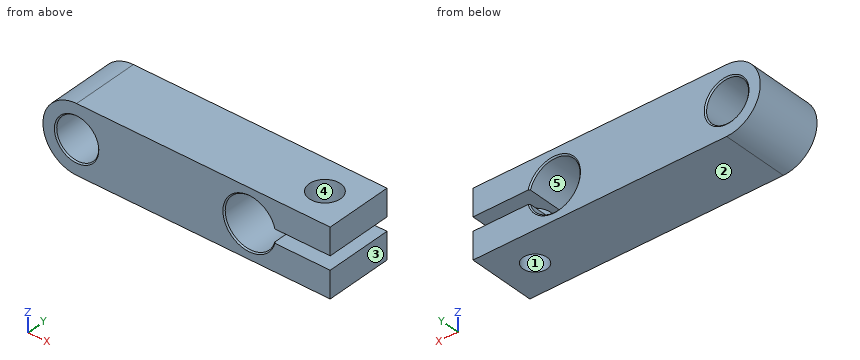
from build123d import *
from OCP.BRepFilletAPI import BRepFilletAPI_MakeChamfer

# Parameters (mm, degrees)
SKETCH1_R                  = 1.9812
SKETCH1_R_2                = 2.38125
BOSS_EXTRUDE1_DEPTH        = 6.35
SKETCH2_W                  = 7.62
SKETCH2_H                  = 1.27
CUT_EXTRUDE1_DEPTH         = 26.532761738
CHAMFER1_SIZE              = 0.127
CHAMFER1_SIZE2             = 0.110399416
F_4_40_TAPPED_HOLE1_REACH  = 27.533
F_4_40_TAPPED_HOLE1_BORE_R = 1.1303
SKETCH5_R                  = 1.4732
CUT_EXTRUDE2_DEPTH         = 2.54


with BuildPart() as part:
    # Sketch1 → Boss-Extrude1 (new body)
    with BuildSketch(Plane(origin=(0, 0, 0), x_dir=(1, 0, 0), z_dir=(0, 1, 0))):
        with BuildLine():
            Line((0, 0), (23.9014, 0))
            Line((23.9014, 0), (23.9014, 6.35))
            Line((23.9014, 6.35), (0, 6.35))
            ThreePointArc((0, 6.35), (-3.175, 3.175), (0, 0))
        make_face()
        with Locations(Location((0, 3.175, 0), (0, 0, 270))):
            Circle(SKETCH1_R, mode=Mode.SUBTRACT)
        with Locations(Location((16.2814, 3.175, 0), (0, 0, 270))):
            Circle(SKETCH1_R_2, mode=Mode.SUBTRACT)
    extrude(amount=BOSS_EXTRUDE1_DEPTH)

    # Sketch2 → Cut-Extrude1 (cut, through all)
    with BuildSketch(Plane(origin=(0, 6.35, 0), x_dir=(1, 0, 0), z_dir=(0, 1, 0))):
        with Locations((20.0914, 3.175)):
            Rectangle(SKETCH2_W, SKETCH2_H)
    extrude(amount=-CUT_EXTRUDE1_DEPTH, mode=Mode.SUBTRACT)

    # Chamfer1: one chamfer whose edges measure the first distance from different faces: ONE call of the kernel's chamfer builder (chamfer() names one face for all edges)
    chamfer1_edges_1 = [part.edges().sort_by_distance(p)[0] for p in [
        (0, 0, -5.1562),
    ]]
    chamfer1_side_1 = [part.faces().sort_by_distance(p)[0] for p in [
        (0, 3.175, -5.1562),
    ]]
    chamfer1_edges_2 = [part.edges().sort_by_distance(p)[0] for p in [
        (0, 6.35, -5.1562),
        (13.90015, 6.35, -3.175),
    ]]
    chamfer1_side_2 = [part.faces().sort_by_distance(p)[0] for p in [
        (10.400868542, 6.35, -3.175),
    ]]
    chamfer1_edges_3 = [part.edges().sort_by_distance(p)[0] for p in [
        (13.90015, 0, -3.175),
    ]]
    chamfer1_side_3 = [part.faces().sort_by_distance(p)[0] for p in [
        (13.90015, 3.175, -3.175),
    ]]
    chamfer1 = BRepFilletAPI_MakeChamfer(part.part.solid().wrapped)
    for e in chamfer1_edges_1:
        chamfer1.Add(CHAMFER1_SIZE, CHAMFER1_SIZE2, e.wrapped, chamfer1_side_1[0].wrapped)  # the first distance lies on this face
    for e in chamfer1_edges_2:
        chamfer1.Add(CHAMFER1_SIZE, CHAMFER1_SIZE2, e.wrapped, chamfer1_side_2[0].wrapped)  # the first distance lies on this face
    for e in chamfer1_edges_3:
        chamfer1.Add(CHAMFER1_SIZE, CHAMFER1_SIZE2, e.wrapped, chamfer1_side_3[0].wrapped)  # the first distance lies on this face
    add(Compound.cast(chamfer1.Shape()), mode=Mode.REPLACE)

    # #4-40 Tapped Hole1 bore → #4-40 Tapped Hole1 (cut, up to next)
    with BuildSketch(Plane(origin=(0, 0, -6.35), x_dir=(-1, 0, 0), z_dir=(0, 0, -1)), mode=Mode.PRIVATE) as f_4_40_tapped_hole1_sk1:
        with Locations((-20.7264, 3.175)):
            Circle(F_4_40_TAPPED_HOLE1_BORE_R)
    f_4_40_tapped_hole1_tool1 = extrude(f_4_40_tapped_hole1_sk1.sketch, amount=-F_4_40_TAPPED_HOLE1_REACH, mode=Mode.PRIVATE) & part.part
    add(f_4_40_tapped_hole1_tool1.solids().sort_by_distance((20.7264, 3.175, -6.35))[0], mode=Mode.SUBTRACT)

    # Sketch5 → Cut-Extrude2 (cut)
    with BuildSketch(Plane.XY):
        with Locations((20.7264, 3.175)):
            Circle(SKETCH5_R)
    extrude(amount=-CUT_EXTRUDE2_DEPTH, mode=Mode.SUBTRACT)


solid = part.part
CAD build for the part. Positions are in the model's coordinates, mm. Face numbers are marked on the shaded views. A direction names the side the tool comes from. Coordinates: 2 decimals unless noted, no trailing zeros. Write each loop counter-clockwise with the first axis right and the second up, starting at its lowest first coordinate (ties: lowest second). Pieces come first, ordered by that corner, then holes. Notation, with made-up numbers: M 13,-34 L 37,-34 A31 cw 37,-6 Z; hole C 6.5,38 d1. An arc over 180 degrees is marked long. Answer as a JSON object with one key per item and string values. Group by question number.
1) Mould opens along X. For the marked faces 1, 2 and 3 say: +X half, -X half, draft (parallel to the pull), parting line (faces both ways), or undercut.
2) Wall check: line 1 (X direction, y = 3.25, z = -4.5); line 2 (Z direction, x = 19, y = 5.5); line 3 (X direction, y = 4.75, z = -4). Give the ranges that are in metal, low to high. Write a range as from..to.
3) Saw through at C-C (y = 4). Give the number of separate pieces and of enclosed holes in the cut face, plus the area to 3 significant figures.
4) Pin check, flat tips, straight feed: pin 1 Ø3 at (y, z) = (3, -3) entering from +X; pin 2 Ø1.8 at (x, y) = (20.73, 3.18) entering from -Z. Stop position of each tip, or through.
5) Tool access for the marked faces 4 and 5: list every direction of +Z, -Z, +X, -X, +Y, -Y with a clear straight run to the whole face (end or side of a thin tool).
6) Saw through at B-B (x = 20). Write the cut outline in (y, z), plus the area to 3 significant figures.
Values follow:
{
 "1": {"face 1": "undercut", "face 2": "draft", "face 3": "+X half"},
 "2": {"line 1": "x = -2.89..-1.47, 1.47..14.3, 18.26..19.6, 21.85..23.9", "line 2": "z = -6.35..-3.81, -2.54..0", "line 3": "x = -3.07..-1.8, 1.8..14.05, 18.52..23.9"},
 "3": {"separate pieces": "3", "enclosed holes": "1", "area": "121 mm2"},
 "4": {"pin 1": "stops at x = 23.9", "pin 2": "passes through"},
 "5": {"face 4": "+Z", "face 5": "+Y, -Y"},
 "6": {"outline": "M 0,-6.35 L 2.31,-6.35 L 2.31,-3.81 L 0,-3.81 Z; M 0,-2.54 L 1.89,-2.54 L 1.89,0 L 0,0 Z; M 4.04,-6.35 L 6.35,-6.35 L 6.35,-3.81 L 4.04,-3.81 Z; M 4.46,-2.54 L 6.35,-2.54 L 6.35,0 L 4.46,0 Z", "area": "21.3 mm2"}
}
